from build123d import *

# Parameters (mm, degrees)
BOSS_EXTRUDE1_DEPTH                            = 5
BOSS_EXTRUDE3_DEPTH                            = 1.5
FILLET1_R                                      = 2
CSK_FOR_M2_FLAT_HEAD_MACHINE_SCREW1_AT_2_COUNT = 2
CSK_FOR_M2_FLAT_HEAD_MACHINE_SCREW1_AT_2_PITCH = 40
CHAMFER1_SIZE                                  = 2


with BuildPart() as part:
    # Sketch1 → Boss-Extrude1 (new body)
    with BuildSketch(Plane(origin=(0, 0, 0), x_dir=(1, 0, 0), z_dir=(0, 1, 0))):
        Polygon((-14.18, 46.928571429), (-14.18, 50), (-17.13, 50), (-17.13, 0), (-14.18, 0), (-14.18, 3.071428571), (-9.703639402, 3.071428571), (-5.570306069, 13.785714286), (-1.78, 13.785714286), (-1.78, 0), (0, 0), (0, 50), (-1.78, 50), (-1.78, 36.214285714), (-5.570306069, 36.214285714), (-9.703639402, 46.928571429), align=None)
        Polygon((-14.18, 4.071428571), (-14.18, 24.5), (-10.389693931, 24.5), (-6.449249487, 14.285714286), (-10.389693931, 4.071428571), align=None, mode=Mode.SUBTRACT)
        Polygon((-10.389693931, 45.928571429), (-6.449249487, 35.714285714), (-10.389693931, 25.5), (-14.18, 25.5), (-14.18, 45.928571429), align=None, mode=Mode.SUBTRACT)
        Polygon((-5.570306069, 14.785714286), (-9.510750513, 25), (-5.570306069, 35.214285714), (-1.78, 35.214285714), (-1.78, 14.785714286), align=None, mode=Mode.SUBTRACT)
    extrude(amount=BOSS_EXTRUDE1_DEPTH)

    # Sketch5 → Boss-Extrude3 (add)
    with BuildSketch(Plane.XZ):
        Polygon((12, -40), (12, -50), (0, -50), (0, 0), (12, 0), (12, -10), (7, -10), (7, -40), align=None)
    extrude(amount=-BOSS_EXTRUDE3_DEPTH)

    # Fillet1
    fillet1_edges = [part.edges().sort_by_distance(p)[0] for p in [
        (12, 0.75, -40),
        (12, 0.75, -50),
        (12, 0.75, 0),
        (12, 0.75, -10),
        (7, 0.75, -10),
        (7, 0.75, -40),
    ]]
    fillet(fillet1_edges, radius=FILLET1_R)

    # Sketch6 → CSK for M2 Flat Head Machine Screw1 (revolve, cut)
    with BuildSketch(Plane(origin=(7, 0, -5), x_dir=(0, 0, -1), z_dir=(1, 0, 0))):
        Polygon((0, 0), (0, 1.5), (1.2, 1.5), (1.2, 1), (2.2, 0), align=None)
    csk_for_m2_flat_head_machine_screw1 = revolve(axis=Axis((7, -6.35, -5), (0, 1, 0)), mode=Mode.SUBTRACT)

    # CSK for M2 Flat Head Machine Screw1 at 2: CSK for M2 Flat Head Machine Screw1 ×2
    with Locations(*[(0, 0, -i * CSK_FOR_M2_FLAT_HEAD_MACHINE_SCREW1_AT_2_PITCH) for i in range(1, CSK_FOR_M2_FLAT_HEAD_MACHINE_SCREW1_AT_2_COUNT)]):
        add(csk_for_m2_flat_head_machine_screw1, mode=Mode.SUBTRACT)

    # Chamfer1
    chamfer1_edges = [part.edges().sort_by_distance(p)[0] for p in [
        (-17.13, 5, -25),
    ]]
    chamfer(chamfer1_edges, length=CHAMFER1_SIZE)


solid = part.part
Verification items for the finished model (mm, model axes). A direction names the side the tool comes from. Coordinates: 2 decimals unless noted, no trailing zeros. Order: outer loops, then holes, each group sorted by start corner. A loop starts at its lowest first (then second) coordinate and runs counter-clockwise, first axis right, second up. Notation, with made-up numbers: (-17, 84) -> (30, 84) arc R26 cw to (30, 120) -> close; hole circle Ø11 at (17.25, -36). An arc over 180 degrees is marked (long way). Use CSV: the item, a comma, the result in double quotes. Start each with the question number.
Q1. Tool access check on faces 5 (the flat face through (-1.78, 2, -43)), 6 (the flat face through (-12, 2, -4.071)), 7 (the cylindrical face through (11.43, 0.76, -40.6)). Record the directions out of +Z, -Z, +X, -X, +Y, -Y that give a thin tool (end or side, any length) a straight path to the whole face; none if there is none.
Q2. Section check D-D, the plane z = -9.5. Record the cut outline in (x, y).
Q3. Section check C-C, the plane x = -11. Record the cut outline in (y, z), and give its area (3 significant figures).
Q4. Section check B-B, the plane x = -2.25. Record the cut outline in (y, z).
Q5. Depth check by flat-ended pin: P1, Ø1.5, axis at y = 2.5, z = -33, coming from the +X side; P2, Ø3, axis at x = -12, y = 3.5, coming from the +Z side; P3, Ø1.9, axis at x = -4, y = 1.5, coming from the -Z side; P4, Ø3, axis at x = -8.5, z = -39.5, coming from the -Y side. Enter the tip coordinate at first touch or a pass-through.
Q6. Draft check along X on faces 1 (the flat face through (-7.513, 2.465, -19.821)), 2 (the flat face through (-14.18, 2, -14)), 3 (the flat face through (-9, 5, -27)), 4 (the cylindrical face through (11.43, 0.76, -0.6)). Enter one of: +X half, -X half, draft (parallel to the pull), parting line (faces both ways), or undercut.
Q7. Section check A-A, the plane y = 2.5. Give the number of separate pieces and of enclosed holes in the cut face, and give its area (3 significant figures).
Q8. Thickness scan on line 1 along Z through (x, y) = (-13.75, 3.55); line 2 along X through (y, z) = (1.55, -10.5); line 3 along X through (y, z) = (1.25, -45). Record the ranges inside material, lowest first.
Returned:
1,face 5,"-Z, +Y, -Y"
1,face 6,"+Y, -Y"
1,face 7,"+X, +Y, -Y"
2,outline,"(-17.13, 0) -> (-14.18, 0) -> (-14.18, 5) -> (-15.13, 5) -> (-17.13, 3) -> close; (-8.3, 0) -> (-7.22, 0) -> (-7.22, 5) -> (-8.3, 5) -> close; (-1.78, 0) -> (11.32, 0) -> (11.32, 1.5) -> (0, 1.5) -> (0, 5) -> (-1.78, 5) -> close"
3,outline,"(0, -46.93) -> (5, -46.93) -> (5, -45.93) -> (0, -45.93) -> close; (0, -25.5) -> (5, -25.5) -> (5, -24.5) -> (0, -24.5) -> close; (0, -4.07) -> (5, -4.07) -> (5, -3.07) -> (0, -3.07) -> close"
3,area,"15.0 mm^2"
4,outline,"(0, -36.21) -> (5, -36.21) -> (5, -35.21) -> (0, -35.21) -> close; (0, -14.79) -> (5, -14.79) -> (5, -13.79) -> (0, -13.79) -> close"
5,P1,"stops at x = 0"
5,P2,"stops at z = -3.07"
5,P3,"stops at z = -36.21"
5,P4,"stops at y = 0"
6,face 1,"undercut"
6,face 2,"undercut"
6,face 3,"draft"
6,face 4,"+X half"
7,separate pieces,"1"
7,enclosed holes,"3"
7,area,"302 mm^2"
8,line 1,"z = -46.93 to -45.93, -25.5 to -24.5, -4.07 to -3.07"
8,line 2,"x = -17.13 to -14.18, -7.91 to -6.84, -1.78 to 0"
8,line 3,"x = -17.13 to -14.18, -10.03 to -8.96, -1.78 to 5.8, 8.2 to 12"
